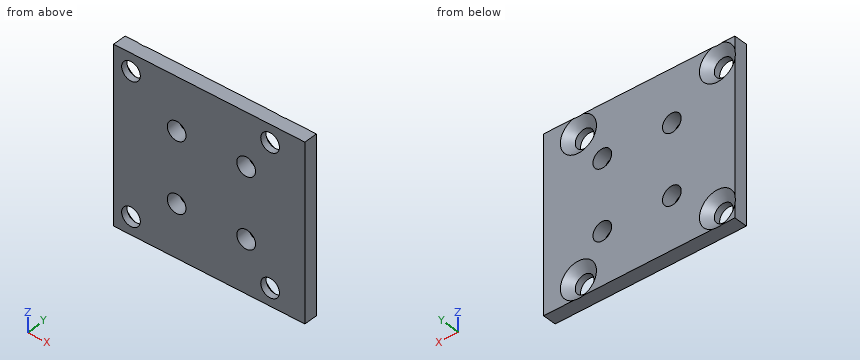
from build123d import *

# Parameters (mm, degrees)
SKETCH1_W            = 43
SKETCH1_H            = 40
BOSS_EXTRUDE1_DEPTH  = 3.125
M4_CLEARANCE_HOLE1_D = 4.3
M4_CLEARANCE_HOLE2_D = 4.3
SKETCH7_W            = 40
SKETCH7_H            = 3.125
BOSS_EXTRUDE2_DEPTH  = 1
CHAMFER1_SIZE        = 2
CHAMFER1_SIZE_2      = 1.678199262


with BuildPart() as part:
    # Sketch1 → Boss-Extrude1 (new body)
    with BuildSketch(Plane(origin=(0, 0, 0), x_dir=(1, 0, 0), z_dir=(0, 1, 0))):
        Rectangle(SKETCH1_W, SKETCH1_H)
    extrude(amount=BOSS_EXTRUDE1_DEPTH)

    # M4 Clearance Hole1 (through all)
    with Locations(Plane(origin=(0, 3.125, 0), x_dir=(1, 0, 0), z_dir=(0, 1, 0))):
        with Locations((-18.5, 16), (13.5, 16), (13.5, -16), (-18.5, -16)):
            Hole(M4_CLEARANCE_HOLE1_D / 2)

    # M4 Clearance Hole2 (through all)
    with Locations(Plane(origin=(0, 3.125, 0), x_dir=(1, 0, 0), z_dir=(0, 1, 0))):
        with Locations((-8, 8), (8, 8), (8, -8), (-8, -8)):
            Hole(M4_CLEARANCE_HOLE2_D / 2)

    # Sketch7 → Boss-Extrude2 (add)
    with BuildSketch(Plane.ZY.offset(21.5)):
        with Locations((0, 1.5625)):
            Rectangle(SKETCH7_W, SKETCH7_H)
    extrude(amount=BOSS_EXTRUDE2_DEPTH)

    # Chamfer1
    # the kernel refuses this chamfer: 2, 1.678199262 mm, written as the material it takes off along each edge
    with BuildSketch(Plane(origin=(-18.5, 3.125, 16), x_dir=(-1, 0, 0), z_dir=(0, 0, 1))) as chamfer1_piece_1:
        Polygon((2.15 + CHAMFER1_SIZE, 0), (2.15, CHAMFER1_SIZE_2), (2.15, 0), align=None)
    revolve(axis=Axis((-18.5, 3.125, 16), (0, -1, 0)), mode=Mode.SUBTRACT)
    with BuildSketch(Plane(origin=(13.5, 3.125, 16), x_dir=(-1, 0, 0), z_dir=(0, 0, 1))) as chamfer1_piece_2:
        Polygon((2.15 + CHAMFER1_SIZE, 0), (2.15, CHAMFER1_SIZE_2), (2.15, 0), align=None)
    revolve(axis=Axis((13.5, 3.125, 16), (0, -1, 0)), mode=Mode.SUBTRACT)
    with BuildSketch(Plane(origin=(13.5, 3.125, -16), x_dir=(-1, 0, 0), z_dir=(0, 0, 1))) as chamfer1_piece_3:
        Polygon((2.15 + CHAMFER1_SIZE, 0), (2.15, CHAMFER1_SIZE_2), (2.15, 0), align=None)
    revolve(axis=Axis((13.5, 3.125, -16), (0, -1, 0)), mode=Mode.SUBTRACT)
    with BuildSketch(Plane(origin=(-18.5, 3.125, -16), x_dir=(-1, 0, 0), z_dir=(0, 0, 1))) as chamfer1_piece_4:
        Polygon((2.15 + CHAMFER1_SIZE, 0), (2.15, CHAMFER1_SIZE_2), (2.15, 0), align=None)
    revolve(axis=Axis((-18.5, 3.125, -16), (0, -1, 0)), mode=Mode.SUBTRACT)


solid = part.part
Can you work these out from the model? Positions are in its coordinate system, mm. Give positions to 0.01 mm unless a question says otherwise; leave off trailing zeros. Loops run counter-clockwise (first coordinate to the right, second up) from the corner with the lowest first, then second, coordinate; pieces in that order, holes last. Notation, with made-up numbers: M -24,54.25 L 34,54.25 A13 cw 34,67.25 Z; hole C 40,46.25 d8. An arc over 180 degrees is marked long. One line per item, written item: value. Start each with the question number.
1) If we section it at C-C, the plane x = -18.5: Write out the boundary of the cut face in (y, z) (3 decimals).
2) I'm going to push flat-ended pins straight in: pin 1 (5 mm diameter, centred on x = 4.5, z = 10.5, fed in from -Y); pin 2 (5 mm diameter, centred on x = -18.5, z = 16, fed in from +Y). Where does each tip first touch, or does it pass through?
3) If we section it at A-A, the plane x = -8: Write out the boundary of the cut face in (y, z) (3 decimals), and give its area (3 significant figures).
4) If I drill on line 1 (X direction, y = 0.5, z = -16); line 2 (Z direction, x = -8, y = 2.6); line 3 (Z direction, x = 13.5, y = 0.4), over which ranges is the centre line in solid material (lowest first)? Write a range as [from, to].
5) If we section it at B-B, the plane z = 16: Write out the boundary of the cut face in (x, y) (3 decimals), and give its area (3 significant figures).
Completed:
1. outline: M 0,-20 L 2.999,-20 L 1.447,-18.15 L 0,-18.15 Z; M 0,-13.85 L 1.447,-13.85 L 3.125,-11.85 L 3.125,11.85 L 1.447,13.85 L 0,13.85 Z; M 0,18.15 L 1.447,18.15 L 2.999,20 L 0,20 Z
2. pin 1: stops at y = 0
2. pin 2: stops at y = 1.74
3. outline: M 0,-20 L 3.125,-20 L 3.125,-10.15 L 0,-10.15 Z; M 0,-5.85 L 3.125,-5.85 L 3.125,5.85 L 0,5.85 Z; M 0,10.15 L 3.125,10.15 L 3.125,20 L 0,20 Z
3. area: 98.1 mm^2
4. line 1: x = [-22.5, -20.65], [-16.35, 11.35], [15.65, 21.5]
4. line 2: z = [-20, -10.15], [-5.85, 5.85], [10.15, 20]
4. line 3: z = [-20, -18.15], [-13.85, 13.85], [18.15, 20]
5. outline: M -22.5,0 L -20.65,0 L -20.65,1.447 L -22.5,2.999 Z; M -16.35,0 L 11.35,0 L 11.35,1.447 L 9.35,3.125 L -14.35,3.125 L -16.35,1.447 Z; M 15.65,0 L 21.5,0 L 21.5,3.125 L 17.65,3.125 L 15.65,1.447 Z
5. area: 104 mm^2
